Part print with two shaded views. Sizes in mm from the minimum x, y, z corner. A direction names the side the tool comes from. Round coordinates to 2 decimals unless told otherwise and drop trailing zeros. Order: outer loops, then holes, each group sorted by start corner. A loop starts at its lowest first (then second) coordinate and runs counter-clockwise, first axis right, second up. Notation, with made-up numbers: (52.25, 72.25) - (83.25, 72.25) arc R21 ccw to (83.25, 83.25) - close; hole circle Ø5 at (8.5, 8). An arc over 180 degrees is marked (long way). Answer as CSV lines item,"result". Start each with the question number.
1. Pin check, flat tips, straight feed: pin 1 Ø0.6 at (y, z) = (30, 8.5) entering from -X; pin 2 Ø4 at (x, y) = (3, 26) entering from +Z; pin 3 Ø1 at (x, y) = (3.5, 27) entering from -Z; pin 4 Ø3 at (x, y) = (15, 29.5) entering from +Z. Stop position of each tip, or through.
2. Band-saw the part on B-B on y = 7.5. List the corners of the cut face in (x, z).
3. Wall check: line 1 along Y through (x, z) = (15, 7.55); line 2 along Y through (x, z) = (13.5, 8); line 3 along X through (y, z) = (3, 4.75). Give the ranges that are in metal, low to high. Write a range as [from, to].
4. Band-saw the part on A-A on y = 29.5. List the corners of the cut face in (x, z), then the cut area to 3 significant figures.
5. Band-saw the part on C-C on x = 14.75. List the corners of the cut face in (y, z).
6. 3-axis set-ups, long thin cutter, end or side, ignore diameter. For the marked faces 1 and 2: which of +Z, -Z, +X, -X, +Y, -Y reach the whole face in a straight line?
7. Band-saw the part on D-D on z = 4.5. List the corners of the cut face in (x, y), then the cut area to 3 significant figures.
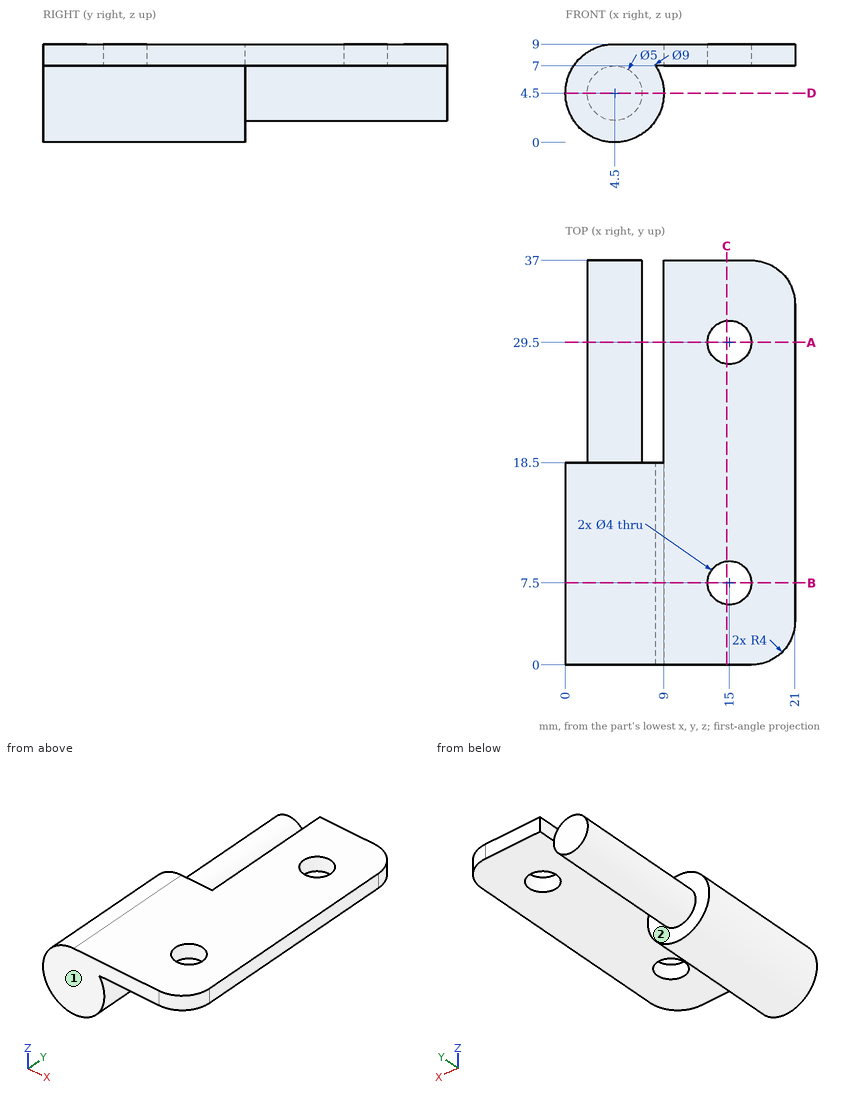
Reply:
1,pin 1,"stops at x = 9"
1,pin 2,"stops at z = 7"
1,pin 3,"stops at z = 2.05"
1,pin 4,"passes through"
2,outline,"(4.5, 9) arc R4.5 ccw (long way) to (8.24, 7) - (13, 7) - (13, 9) - close; (17, 7) - (21, 7) - (21, 9) - (17, 9) - close"
3,line 1,"y = [0, 5.5], [9.5, 27.5], [31.5, 37]"
3,line 2,"y = [0, 6.18], [8.82, 28.18], [30.82, 37]"
3,line 3,"x = [0.01, 8.99]"
4,outline,"circle Ø5 at (4.5, 4.5); (9, 7) - (13, 7) - (13, 9) - (9, 9) - close; (17, 7) - (21, 7) - (21, 9) - (17, 9) - close"
4,area,"35.6 mm2"
5,outline,"(0, 7) - (5.52, 7) - (5.52, 9) - (0, 9) - close; (9.48, 7) - (27.52, 7) - (27.52, 9) - (9.48, 9) - close; (31.48, 7) - (37, 7) - (37, 9) - (31.48, 9) - close"
6,face 1,"+Z, -Z, +X, -X, -Y"
6,face 2,"+Y"
7,outline,"(0, 0) - (9, 0) - (9, 18.5) - (7, 18.5) - (7, 37) - (2, 37) - (2, 18.5) - (0, 18.5) - close"
7,area,"259 mm2"
